from build123d import *

# Parameters (mm, degrees)
SKETCH_1_W               = 120
SKETCH_1_H               = 80
EXTRUDE_1_DEPTH          = 20
CUT_EXTRUDE_1_DEPTH      = 146.602197786
CUT_EXTRUDE_1_DEPTH_BACK = 146.602197786
SKETCH_3_W               = 72
SKETCH_3_H               = 30
EXTRUDE_2_DEPTH          = 90
EXTRUDE_3_DEPTH          = 50
FILLET_1_R               = 15
CUT_EXTRUDE_2_DEPTH      = 171.293863659
CUT_EXTRUDE_2_DEPTH_BACK = 171.293863659
SKETCH_5_W               = 40
SKETCH_5_H               = 20


with BuildPart() as part:
    # 草图1 → 凸台-拉伸1 (new body)
    with BuildSketch(Plane(origin=(0, 0, 0), x_dir=(1, 0, 0), z_dir=(0, 1, 0))):
        with Locations((60, -40)):
            Rectangle(SKETCH_1_W, SKETCH_1_H)
    extrude(amount=EXTRUDE_1_DEPTH)

    # 草图2 → 切除-拉伸1 (cut, two sides: drawn at the far end of the back side and taken through both)
    with BuildSketch(Plane.XY.offset(80).offset(-CUT_EXTRUDE_1_DEPTH_BACK)):
        Polygon((60, 0), (105, 0), (96, 9), (57.005784519, 9), (24, 9), (15, 0), align=None)
    extrude(amount=CUT_EXTRUDE_1_DEPTH + CUT_EXTRUDE_1_DEPTH_BACK, mode=Mode.SUBTRACT)

    # 草图3 → 凸台-拉伸2 (add)
    with BuildSketch(Plane(origin=(0, 20, 0), x_dir=(1, 0, 0), z_dir=(0, 1, 0))):
        with Locations((60, -15)):
            Rectangle(SKETCH_3_W, SKETCH_3_H)
    extrude(amount=EXTRUDE_2_DEPTH)

    # 草图3<3> → 凸台-拉伸3 (add)
    with BuildSketch(Plane(origin=(0, 20, 0), x_dir=(1, 0, 0), z_dir=(0, 1, 0))):
        with BuildLine():
            Line((80, -30), (60, -30))
            Line((60, -30), (49.673358607, -30))
            Line((49.673358607, -30), (40, -30))
            Line((40, -30), (35, -30))
            ThreePointArc((35, -30), (60, -55), (85, -30))
            Line((85, -30), (80, -30))
        make_face()
    extrude(amount=EXTRUDE_3_DEPTH)

    # 圆角1
    fillet_1_edges = [part.edges().sort_by_distance(p)[0] for p in [
        (96, 110, 15),
        (24, 110, 15),
    ]]
    fillet(fillet_1_edges, radius=FILLET_1_R)

    # 草图5 → 切除-拉伸2 (cut, two sides: drawn at the far end of the back side and taken through both)
    with BuildSketch(Plane.XY.offset(30).offset(-CUT_EXTRUDE_2_DEPTH_BACK)):
        with Locations((60, 90)):
            Rectangle(SKETCH_5_W, SKETCH_5_H)
    extrude(amount=CUT_EXTRUDE_2_DEPTH + CUT_EXTRUDE_2_DEPTH_BACK, mode=Mode.SUBTRACT)


solid = part.part
Can you work these out from the model? Positions are in its coordinate system, mm. A direction names the side the tool comes from. Round coordinates to 2 decimals unless told otherwise and drop trailing zeros. Order: outer loops, then holes, each group sorted by start corner. A loop starts at its lowest first (then second) coordinate and runs counter-clockwise, first axis right, second up. Notation, with made-up numbers: M 76,70.25 L 97,70.25 A7 ccw 97,80.25 Z; hole C 25,31.5 d9. An arc over 180 degrees is marked long. Use a Markdown table: item, result.
1) Imagine slicing it at D-D (y = 91). List the corners of the cut face in (x, z) for me.
Geometry says:
| item | result |
|---|---|
| outline | M 24,0 L 40,0 L 40,30 L 24,30 Z; M 80,0 L 96,0 L 96,30 L 80,30 Z |
2) Imagine slicing it at C-C (z = 22). List the corners of the cut face in (x, y) for me, then the cut area to 3 significant figures.
Geometry says:
| item | result |
|---|---|
| outline | M 0,0 L 15,0 L 24,9 L 96,9 L 105,0 L 120,0 L 120,20 L 96,20 L 96,95 A15 ccw 81,110 L 39,110 A15 ccw 24,95 L 24,20 L 0,20 Z; hole M 40,80 L 80,80 L 80,100 L 40,100 Z |
| area | 7,250 mm² |
3) I'm going to push flat-ended pins straight in: P1, Ø12, axis at x = 94.5, y = 96, coming from the +Z side; P2, Ø15, axis at x = 57, z = 12.5, coming from the -Y side; P3, Ø2, axis at x = 36.5, y = 42, coming from the +Z side. Where does each tip first touch, or does it pass through?
Geometry says:
| item | result |
|---|---|
| P1 | stops at z = 30 |
| P2 | stops at y = 9 |
| P3 | stops at z = 40.9 |
4) Imagine slicing it at B-B (x = 61). List the corners of the cut face in (y, z) for me, then the cut area to 3 significant figures.
Geometry says:
| item | result |
|---|---|
| outline | M 9,0 L 80,0 L 80,30 L 70,30 L 70,54.98 L 20,54.98 L 20,80 L 9,80 Z; M 100,0 L 110,0 L 110,30 L 100,30 Z |
| area | 4,230 mm² |
5) On a 3-axis mill with a long thin cutter (end or side, diameter ignored), from which of +Z, -Z, +X, -X, +Y, -Y can I reach the whole of each face in a straight line? I mean faces 1 (the face through (60, 70, 40)), 2 (the face through (59.45, 44.65, 54.994)), 3 (the face through (40, 90, 15)). Say none if no direction works.
Geometry says:
| item | result |
|---|---|
| face 1 | +Z, +X, -X, +Y |
| face 2 | +Z, +Y |
| face 3 | +Z, -Z |
6) Imagine slicing it at A-A (y = 7). List the corners of the cut face in (x, z) for me.
Geometry says:
| item | result |
|---|---|
| outline | M 0,0 L 22,0 L 22,80 L 0,80 Z; M 98,0 L 120,0 L 120,80 L 98,80 Z |
7) If I drill on line 1 along Y through (x, z) = (53.5, 19); line 2 along Y through (x, z) = (37.5, 52); line 3 along Y through (x, z) = (6, 71.5), over which ranges is the centre line in solid material (lowest first)?
Geometry says:
| item | result |
|---|---|
| line 1 | y = 9 to 80, 100 to 110 |
| line 2 | y = 9 to 20 |
| line 3 | y = 0 to 20 |
